```python
from build123d import *

# Parameters (mm, degrees)
F0_R     = 11.1125
F1_DEPTH = 25.4
F2_R     = 15.24
F3_DEPTH = 1.27
F4_W     = 53.34
F4_H     = 15.24
F5_DEPTH = 1.016


with BuildPart() as f1:
    # F0 (on Top) → F1 (new body)
    with BuildSketch(Plane.XY):
        with BuildLine():
            ThreePointArc((-31.75, 16.51), (-20.075667, 11.674333), (-15.24, 0))
            ThreePointArc((-15.24, 0), (0, -15.24), (15.24, 0))
            ThreePointArc((15.24, 0), (20.075667, 11.674333), (31.75, 16.51))
            Line((31.75, 16.51), (31.75, 19.05))
            Line((31.75, 19.05), (-31.75, 19.05))
            Line((-31.75, 19.05), (-31.75, 16.51))
        make_face()
        Circle(F0_R, mode=Mode.SUBTRACT)
    extrude(amount=F1_DEPTH)

    # F2 (on face) → F3 (join)
    with BuildSketch(Plane(origin=(0, 0, 0), x_dir=(1, 0, 0), z_dir=(0, 0, -1))):
        Circle(F2_R)
    extrude(amount=-F3_DEPTH)

    # F4 (on face) → F5 (cut)
    with BuildSketch(Plane(origin=(0, 19.05, 0), x_dir=(-1, 0, 0), z_dir=(0, 1, 0))):
        with Locations((0, 12.7)):
            Rectangle(F4_W, F4_H)
    extrude(amount=-F5_DEPTH, mode=Mode.SUBTRACT)


solid = f1.part
```
Part model, mm, in its own coordinate system. A direction names the side the tool comes from. Round coordinates to 2 decimals unless told otherwise and drop trailing zeros. Order: outer loops, then holes, each group sorted by start corner. A loop starts at its lowest first (then second) coordinate and runs counter-clockwise, first axis right, second up. Notation, with made-up numbers: M 23.25,-23 L 33.25,-23 A30 cw 33.25,12 Z; hole C 12.25,62.5 d9. An arc over 180 degrees is marked long. Answer in a Markdown table with one row per item. Add a question column.
Q1. Cut at D-D on x = 16.5. Give the cut face in (y, z), and give its area (3 significant figures).
Q2. Pin check, flat tips, straight feed: pin 1 (6 mm diameter, centred on y = 6, z = 19, fed in from +X); pin 2 (4 mm diameter, centred on x = -15.5, z = 8.5, fed in from -Y); pin 3 (1.5 mm diameter, centred on x = -1, y = -1, fed in from +Z). Stop position of each tip, or through.
Q3. 3-axis set-ups, long thin cutter, end or side, ignore diameter. For faces 5 (the face through (-20.2, 11.8, 12.5)), 6 (the face through (10.6, 3.34, 13.17)): which of +Z, -Z, +X, -X, +Y, -Y reach the whole face in a straight line?
Q4. Wall check: L1, parallel to Y at x = 0, z = 8.5; L2, parallel to X at y = 0, z = 8; L3, parallel to Z at x = -6, y = -9. Give the ranges that are in metal, low to high. Write a range as from..to.
Q5. Mould opens along Z. For faces 1 (the face through (0, 19.05, 4)), 2 (the face through (0, 0, 1.27)), 3 (the face through (0, 6, 0)), 4 (the face through (0, 18.034, 13)) say: +Z half, -Z half, draft (parallel to the pull), parting line (faces both ways), or undercut.
Q6. Cut at C-C on y = 4. Give the cut face in (x, z), and give its area (3 significant figures).
Q7. Cut at B-B on x = 0. Give the cut face in (y, z).
Established:
| question | item | result |
|---|---|---|
| 1 | outline | M 6.33,0 L 19.05,0 L 19.05,5.08 L 18.03,5.08 L 18.03,20.32 L 19.05,20.32 L 19.05,25.4 L 6.33,25.4 Z |
| 1 | area | 308 mm2 |
| 2 | pin 1 | stops at x = 17.91 |
| 2 | pin 2 | stops at y = -7.07 |
| 2 | pin 3 | stops at z = 1.27 |
| 3 | face 5 | +Z, -Z, -X, -Y |
| 3 | face 6 | +Z |
| 4 | L1 | y = -15.24..-11.11, 11.11..18.03 |
| 4 | L2 | x = -15.24..-11.11, 11.11..15.24 |
| 4 | L3 | z = 0..1.27 |
| 5 | face 1 | draft |
| 5 | face 2 | +Z half |
| 5 | face 3 | -Z half |
| 5 | face 4 | undercut |
| 6 | outline | M -15.73,0 L 15.73,0 L 15.73,25.4 L 10.37,25.4 L 10.37,1.27 L -10.37,1.27 L -10.37,25.4 L -15.73,25.4 Z |
| 6 | area | 299 mm2 |
| 7 | outline | M -15.24,0 L 19.05,0 L 19.05,5.08 L 18.03,5.08 L 18.03,20.32 L 19.05,20.32 L 19.05,25.4 L 11.11,25.4 L 11.11,1.27 L -11.11,1.27 L -11.11,25.4 L -15.24,25.4 Z |
